from build123d import *

# Parameters (mm, degrees)
F0_W     = 530
F0_H     = 547
F0_W_2   = 410
F0_H_2   = 427
F1_DEPTH = 60
F2_W     = 60
F2_H     = 60
F3_DEPTH = 300
F4_W     = 530
F4_H     = 547
F4_W_2   = 410
F4_H_2   = 427
F5_DEPTH = 60
F6_W     = 60
F6_H     = 60
F7_DEPTH = 50


with BuildPart() as f1:
    # F0 (on Top) → F1 (new body)
    with BuildSketch(Plane.XY):
        Rectangle(F0_W, F0_H)
        Rectangle(F0_W_2, F0_H_2, mode=Mode.SUBTRACT)
    extrude(amount=F1_DEPTH)

    # F2 (on face) → F3 (join)
    with BuildSketch(Plane(origin=(0, 0, 0), x_dir=(1, 0, 0), z_dir=(0, 0, -1))):
        with Locations((-235, 243.5)):
            Rectangle(F2_W, F2_H)
        with Locations((235, 243.5)):
            Rectangle(F2_W, F2_H)
        with Locations((-235, -243.5)):
            Rectangle(F2_W, F2_H)
        with Locations((235, -243.5)):
            Rectangle(F2_W, F2_H)
    extrude(amount=F3_DEPTH)

    # F4 (on face) → F5 (join)
    with BuildSketch(Plane(origin=(0, 0, -300), x_dir=(1, 0, 0), z_dir=(0, 0, -1))):
        Rectangle(F4_W, F4_H)
        Rectangle(F4_W_2, F4_H_2, mode=Mode.SUBTRACT)
    extrude(amount=F5_DEPTH)

    # F6 (on face) → F7 (join)
    with BuildSketch(Plane(origin=(0, 0, -360), x_dir=(1, 0, 0), z_dir=(0, 0, -1))):
        with Locations((-235, 243.5)):
            Rectangle(F6_W, F6_H)
        with Locations((235, 243.5)):
            Rectangle(F6_W, F6_H)
        with Locations((-235, -243.5)):
            Rectangle(F6_W, F6_H)
        with Locations((235, -243.5)):
            Rectangle(F6_W, F6_H)
    extrude(amount=F7_DEPTH)


solid = f1.part
Model file for the job. Use its own axes, mm. A direction names the side the tool comes from. Give positions to 0.01 mm unless a question says otherwise; leave off trailing zeros. Order: outer loops, then holes, each group sorted by start corner. A loop starts at its lowest first (then second) coordinate and runs counter-clockwise, first axis right, second up. Notation, with made-up numbers: (4.5, -19.75) - (37.5, -19.75) arc R23 ccw to (37.5, 15.25) - close; hole circle Ø7 at (-7, 30.5). An arc over 180 degrees is marked (long way). One line per item, written item: value.
Item 1: Wall check: line 1 (Z direction, x = -56, y = -221); line 2 (X direction, y = 244.5, z = -133.5). Give the ranges that are in metal, low to high.
Response values:
line 1: -360 to -300, 0 to 60
line 2: -265 to -205, 205 to 265
Item 2: Pin check, flat tip, straight feed: pin 1 Ø18 at (x, y) = (237, -31.5) entering from -Z. Stop position of the tip, or through.
Response values:
pin 1: z = -360
Item 3: Slice it at C-C (z = -313). List the corners of the cut face in (x, y), then the cut area to 3 significant figures.
Response values:
outline: (-265, -273.5) - (265, -273.5) - (265, 273.5) - (-265, 273.5) - close; hole (-205, -213.5) - (205, -213.5) - (205, 213.5) - (-205, 213.5) - close
area: 115,000 mm2
Item 4: Two-plate mould, pull along Z, no slides. Class faces 5 (the flat face through (-3, -244, -360)), 6 (the flat face through (-235, -213.5, -148)), 7 (the flat face through (-205, -3, 30)): released by +Z, released by -Z, zero draft, split by the parting line, or undercut.
Response values:
face 5: released by -Z
face 6: undercut
face 7: zero draft
Item 5: Slice it at B-B (y = 100). List the corners of the cut face in (x, z).
Response values:
outline: (-265, -360) - (-205, -360) - (-205, -300) - (-265, -300) - close; (-265, 0) - (-205, 0) - (-205, 60) - (-265, 60) - close; (205, -360) - (265, -360) - (265, -300) - (205, -300) - close; (205, 0) - (265, 0) - (265, 60) - (205, 60) - close
Item 6: Tool access for faces 1 (the flat face through (205, -243, -148)), 2 (the flat face through (235, 3, 0)), 3 (the flat face through (-3, 213.5, -330)), 4 (the flat face through (-205, -243, -385)): list every direction of +Z, -Z, +X, -X, +Y, -Y with a clear straight run to the whole face (end or side of a thin tool).
Response values:
face 1: +Y, -Y
face 2: +X, -X
face 3: +Z, -Z
face 4: -Z, +Y, -Y
Item 7: Slice it at A-A (x = 164.5). List the corners of the cut face in (y, z), then the cut area to 3 significant figures.
Response values:
outline: (-273.5, -360) - (-213.5, -360) - (-213.5, -300) - (-273.5, -300) - close; (-273.5, 0) - (-213.5, 0) - (-213.5, 60) - (-273.5, 60) - close; (213.5, -360) - (273.5, -360) - (273.5, -300) - (213.5, -300) - close; (213.5, 0) - (273.5, 0) - (273.5, 60) - (213.5, 60) - close
area: 14,400 mm2
